The listing builds one solid part. Answer for the finished solid, in the listing's coordinates (mm). Coordinates: 2 decimals unless noted, no trailing zeros. Loops run counter-clockwise (first coordinate to the right, second up) from the corner with the lowest first, then second, coordinate; pieces in that order, holes last. Notation, with made-up numbers: M 87,36 L 101,36 A31 cw 101,67 Z; hole C 50.25,-30.75 d10. An arc over 180 degrees is marked long. Return JSON: item names as keys, results as strings. Group by question number.
1. Straight lines are drawn through the part: L1, parallel to X at y = 6.95, z = 120; L2, parallel to Y at x = 7.75, z = 203; L3, parallel to X at y = 7.25, z = 134.5. For each, find the intervals that lie inside material, in ascending order. Write a range as from..to.
2. Section B-B (y = 6.5) is taken. Count the separate pieces of the cut face and the enclosed holes in it, then the cut area to 3 significant figures.
3. Given P1, Ø3, axis at x = 1, z = -161.5, coming from the +Y side; P2, Ø3, axis at x = 0, z = 320, coming from the +Y side; P3, Ø5, axis at y = 3, z = 217.5, coming from the +X side; P4, Ø1.5, axis at y = 3, z = -73, coming from the +X side, each flat-ended and moving along its own axis, determine where each tip first touches the part or whether it passes through.
4. Section A-A (z = -145) is taken. Write down the section's boundary in (x, y) (3 decimals).
```python
from build123d import *

# Parameters (mm, degrees)
BOSS_EXTRUDE1_DEPTH     = 335
CUT_EXTRUDE1_DEPTH      = 336.281493674
CUT_EXTRUDE1_DEPTH_BACK = 336.281493674
SKETCH4_W               = 0.254
SKETCH4_H               = 0.381
LPATTERN2_COUNT         = 17
LPATTERN2_PITCH         = 40
CUT_EXTRUDE2_DEPTH      = 336.268146414
CUT_EXTRUDE2_DEPTH_BACK = 336.268146414
SKETCH9_W               = 20.4
SKETCH9_H               = 111.2
SKETCH10_R              = 5.61975
CUT_EXTRUDE3_DEPTH      = 3.96875
F_1_4_CLEARANCE_HOLE1_D = 6.7564
LPATTERN3_COUNT         = 7
LPATTERN3_PITCH         = 80


with BuildPart() as part:
    # Sketch1 → Boss-Extrude1 (new, symmetric)
    with BuildSketch(Plane.XY):
        with BuildLine():
            Line((-7.925, 9.2), (-5.8, 9.2))
            Line((-5.8, 9.2), (-5.282234843, 8.7))
            Line((-5.282234843, 8.7), (5.282234843, 8.7))
            Line((5.282234843, 8.7), (5.8, 9.2))
            Line((5.8, 9.2), (7.925, 9.2))
            ThreePointArc((7.925, 9.2), (10.2, 6.925), (7.925, 4.65))
            Line((7.925, 4.65), (4.45, 4.65))
            Line((4.45, 4.65), (4.45, 3.360918321))
            Line((4.45, 3.360918321), (7.246, 1.746646968))
            ThreePointArc((7.246, 1.746646968), (7.431940905, 1.560706063), (7.5, 1.306706063))
            Line((7.5, 1.306706063), (7.5, 0.254))
            ThreePointArc((7.5, 0.254), (7.425605122, 0.074394878), (7.246, 0))
            Line((7.246, 0), (-7.246, 0))
            ThreePointArc((-7.246, 0), (-7.425605122, 0.074394878), (-7.5, 0.254))
            Line((-7.5, 0.254), (-7.5, 1.306706063))
            ThreePointArc((-7.5, 1.306706063), (-7.431940905, 1.560706063), (-7.246, 1.746646968))
            Line((-7.246, 1.746646968), (-4.45, 3.360918321))
            Line((-4.45, 3.360918321), (-4.45, 4.65))
            Line((-4.45, 4.65), (-7.925, 4.65))
            ThreePointArc((-7.925, 4.65), (-10.2, 6.925), (-7.925, 9.2))
        make_face()
    extrude(amount=BOSS_EXTRUDE1_DEPTH, both=True)

    # Sketch4 → Cut-Extrude1 (cut, two sides: drawn at the far end of the back side and taken through both)
    with BuildSketch(Plane.XY.offset(-CUT_EXTRUDE1_DEPTH_BACK)):
        with Locations((7.373, 0.8255)):
            Rectangle(SKETCH4_W, SKETCH4_H)
    extrude(amount=CUT_EXTRUDE1_DEPTH + CUT_EXTRUDE1_DEPTH_BACK, mode=Mode.SUBTRACT)

    # Sketch2 → Cut-Revolve1 (revolve, cut)
    with BuildSketch(Plane(origin=(0, 0, 0), x_dir=(0, 0, -1), z_dir=(1, 0, 0)), mode=Mode.PRIVATE) as cut_revolve1_sk:
        Polygon((-323, 8.7), (-323, 4.7), (-321.75, 4.7), (-321.75, 0), (-320, 0), (-320, 8.7), (-320, 9.2), (-323, 9.2), align=None)
    cut_revolve1 = revolve(cut_revolve1_sk.sketch.rotate(Axis((0, 0, 320), (0, 1, 0)), 180), axis=Axis((0, 0, 320), (0, 1, 0)), mode=Mode.SUBTRACT)

    # LPattern2: Cut-Revolve1 ×17
    with Locations(*[(0, 0, -i * LPATTERN2_PITCH) for i in range(1, LPATTERN2_COUNT)]):
        add(cut_revolve1, mode=Mode.SUBTRACT)

    # Sketch9 → Cut-Extrude2 (cut, two sides: drawn at the far end of the back side and taken through both)
    with BuildSketch(Plane(origin=(0, 8.7, 0), x_dir=(1, 0, 0), z_dir=(0, 1, 0)).offset(-CUT_EXTRUDE2_DEPTH_BACK)):
        with Locations((0, 279.4)):
            Rectangle(SKETCH9_W, SKETCH9_H)
    extrude(amount=CUT_EXTRUDE2_DEPTH + CUT_EXTRUDE2_DEPTH_BACK, mode=Mode.SUBTRACT)

    # Sketch10 → Cut-Extrude3 (cut)
    with BuildSketch(Plane(origin=(0, 8.7, 0), x_dir=(1, 0, 0), z_dir=(0, 1, 0))):
        with Locations(Location((0, 200, 0), (0, 0, 270))):
            Circle(SKETCH10_R)
    cut_extrude3 = extrude(amount=-CUT_EXTRUDE3_DEPTH, mode=Mode.SUBTRACT)

    # 1/4 Clearance Hole1 (through all)
    with Locations(Plane(origin=(0, 4.73125, 0), x_dir=(1, 0, 0), z_dir=(0, 1, 0))):
        with Locations((0, 200)):
            f_1_4_clearance_hole1 = Hole(F_1_4_CLEARANCE_HOLE1_D / 2)

    # LPattern3: Cut-Extrude3, 1/4 Clearance Hole1 ×7
    with Locations(*[(0, 0, i * LPATTERN3_PITCH) for i in range(1, LPATTERN3_COUNT)]):
        add(cut_extrude3, mode=Mode.SUBTRACT)
        add(f_1_4_clearance_hole1, mode=Mode.SUBTRACT)


solid = part.part
```
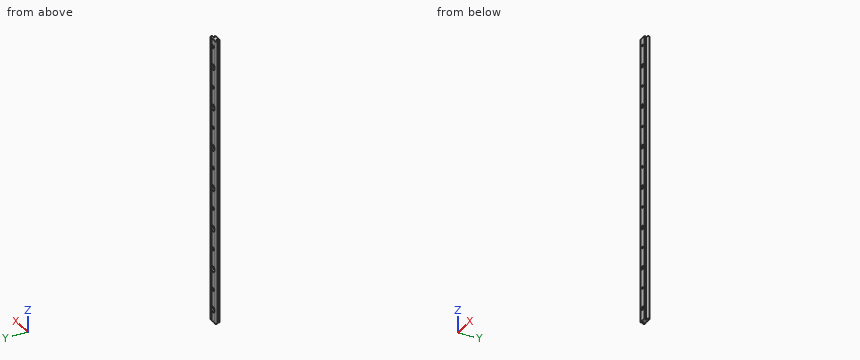
Worked out:
{
 "1": {"L1": "-10.2..-5.62, 5.62..10.2", "L2": "4.65..9.2", "L3": "-10.18..10.18"},
 "2": {"separate pieces": "1", "enclosed holes": "14", "area": "10,500 mm^2"},
 "3": {"P1": "y = 8.7", "P2": "through", "P3": "x = 9.7", "P4": "x = 6.37"},
 "4": {"outline": "M -7.925,4.65 L -4.45,4.65 L -4.45,3.361 L -7.246,1.747 A0.508 ccw -7.5,1.307 L -7.5,0.254 A0.254 ccw -7.246,0 L 7.246,0 A0.254 ccw 7.5,0.254 L 7.5,0.635 L 7.246,0.635 L 7.246,1.016 L 7.5,1.016 L 7.5,1.307 A0.508 ccw 7.246,1.747 L 4.45,3.361 L 4.45,4.65 L 7.925,4.65 A2.275 ccw 7.925,9.2 L 5.8,9.2 L 5.282,8.7 L -5.282,8.7 L -5.8,9.2 L -7.925,9.2 A2.275 ccw Z"}
}
